from build123d import *

# Parameters (mm, degrees)
BOSS_EXTRUDE1_DEPTH        = 6
M16X1_5_TAPPED_HOLE1_D     = 14.5
M16X1_5_TAPPED_HOLE1_DEPTH = 39.5
M16X1_5_TAPPED_HOLE1_TIP   = 4.356239488


with BuildPart() as part:
    # Sketch1 → Boss-Extrude1 (new body)
    with BuildSketch(Plane(origin=(0, 0, 0), x_dir=(1, 0, 0), z_dir=(0, 1, 0))):
        Polygon((6.92820323, 12), (-6.92820323, 12), (-13.856406461, 0), (-6.92820323, -12), (6.92820323, -12), (13.856406461, 0), align=None)
    extrude(amount=BOSS_EXTRUDE1_DEPTH)

    # Sketch2 → Cut-Revolve1 (revolve, cut)
    with BuildSketch(Plane.XY):
        Polygon((-13.856406461, 0), (-10.356406461, 0), (-13.856406461, 0.460783742), align=None)
        Polygon((-13.856406461, 6), (-10.356406461, 6), (-13.856406461, 5.539216258), align=None)
    revolve(axis=Axis((0, 0, 0), (0, 1, 0)), mode=Mode.SUBTRACT)

    # M16x1.5 Tapped Hole1
    with Locations(Plane(origin=(0, 6, 0), x_dir=(1, 0, 0), z_dir=(0, 1, 0))):
        with Locations((0, 0)):
            Hole(M16X1_5_TAPPED_HOLE1_D / 2, depth=M16X1_5_TAPPED_HOLE1_DEPTH)
            with Locations((0, 0, -(M16X1_5_TAPPED_HOLE1_DEPTH + M16X1_5_TAPPED_HOLE1_TIP / 2))):  # 118° drill point
                Cone(0, M16X1_5_TAPPED_HOLE1_D / 2, M16X1_5_TAPPED_HOLE1_TIP, mode=Mode.SUBTRACT)


solid = part.part
Work out the finished part from the listing and answer in its coordinate system (mm). Round coordinates to 2 decimals unless told otherwise and drop trailing zeros. Loops run counter-clockwise (first coordinate to the right, second up) from the corner with the lowest first, then second, coordinate; pieces in that order, holes last. Notation, with made-up numbers: (-8.5, -36.75) - (11.5, -36.75) arc R29 cw to (11.5, -9.75) - close; hole circle Ø10 at (55, 36). An arc over 180 degrees is marked (long way). Use one line per item in the form item = value. Start each with the question number.
(1) Flat-ended cylindrical pins translate along their axes: P1, Ø1, axis at y = 3.5, z = 3.5, coming from the -X side; P2, Ø1.5, axis at y = 0.5, z = -6.5, coming from the +X side. Find the tip coordinate at first contact, or state that the pin passes through.
(2) Consider line 1 (Z direction, x = 0, y = 3.35); line 2 (X direction, y = 4.7, z = 2.5); line 3 (Z direction, x = -5.75, y = 3.2). Determine where each line is inside the solid, lowest interval first.
(3) Determine the mould class of faces 1 (the face through (10.344, 2.961, 6.084)), 2 (the face through (-3.35, 2.96, 6.43)), 3 (the face through (-10.09, 0.03, 3.18)) for opening direction Z: +Z half, -Z half, draft (parallel to the pull), parting line (faces both ways), or undercut.
(4) Find section B-B on x = 0. Determine the outline of the cut face in (y, z).
(5) Find section A-A on y = 2.2. Determine the outline of the cut face in (x, z), and give its area (3 significant figures).
Answer list:
q1.P1 = -12.12
q1.P2 = 10.54
q2.line_1 = -12 to -7.25, 7.25 to 12
q2.line_2 = -12.41 to -6.81, 6.81 to 12.41
q2.line_3 = -12 to -4.42, 4.42 to 12
q3.face_1 = +Z half
q3.face_2 = undercut
q3.face_3 = parting line
q4.outline = (0, -10.36) - (0.22, -12) - (5.78, -12) - (6, -10.36) - (6, -7.25) - (0, -7.25) - close; (0, 7.25) - (6, 7.25) - (6, 10.36) - (5.78, 12) - (0.22, 12) - (0, 10.36) - close
q5.outline = (-13.86, 0) - (-6.93, -12) - (6.93, -12) - (13.86, 0) - (6.93, 12) - (-6.93, 12) - close; hole circle Ø14.5 at (0, 0)
q5.area = 334 mm^2
